```python
from build123d import *

# Parameters (mm, degrees)
EXTRUDE_START   = 4.5
EXTRUDE_1_DEPTH = 3
SKETCH_3_R      = 2.5
EXTRUDE_2_DEPTH = 4.5
SKETCH_6_R      = 3
EXTRUDE_3_DEPTH = 0.5
FILLET_1_R      = 3


with BuildPart() as part:
    # Эскиз2 → Бобышка-Вытянуть1 (new body)
    with BuildSketch(Plane.XY.offset(EXTRUDE_START)):
        with BuildLine():
            ThreePointArc((9, 5.196152423), (0, 0), (9, -5.196152423))
            ThreePointArc((9, -5.196152423), (12, -4.392304845), (15, -5.196152423))
            ThreePointArc((15, -5.196152423), (24, 0), (15, 5.196152423))
            ThreePointArc((15, 5.196152423), (12, 4.392304845), (9, 5.196152423))
        make_face()
    extrude(amount=EXTRUDE_1_DEPTH)

    # Эскиз3 → Бобышка-Вытянуть2 (add)
    with BuildSketch(Plane(origin=(0, 0, 4.5), x_dir=(-1, 0, 0), z_dir=(0, 0, -1))):
        with Locations(Location((-18, 0, 0), (0, 0, 180))):
            Circle(SKETCH_3_R)
        with Locations(Location((-6, 0, 0), (0, 0, 180))):
            Circle(SKETCH_3_R)
    extrude(amount=EXTRUDE_2_DEPTH)

    # Эскиз6 → Бобышка-Вытянуть3 (add)
    with BuildSketch(Plane(origin=(0, 0, 4.5), x_dir=(-1, 0, 0), z_dir=(0, 0, -1))):
        with Locations(Location((-18, 0, 0), (0, 0, 180))):
            Circle(SKETCH_6_R)
        with Locations(Location((-6, 0, 0), (0, 0, 180))):
            Circle(SKETCH_6_R)
    extrude(amount=EXTRUDE_3_DEPTH)

    # Скругление1
    fillet_1_edges = [part.edges().sort_by_distance(p)[0] for p in [
        (0, 0, 7.5),
        (12, 4.392304845, 7.5),
        (24, 0, 7.5),
        (12, -4.392304845, 7.5),
    ]]
    fillet(fillet_1_edges, radius=FILLET_1_R - 0.0001)  # a hair under: the kernel refuses the full size


solid = part.part
```
For this review, take the finished solid that the model builds, in its own axes (mm). A direction names the side the tool comes from. Round coordinates to 2 decimals unless told otherwise and drop trailing zeros. Write each loop counter-clockwise with the first axis right and the second up, starting at its lowest first coordinate (ties: lowest second). Pieces come first, ordered by that corner, then holes. Notation, with made-up numbers: (-5.5, 28.25) -> (8.5, 28.25) arc R21 ccw to (8.5, 66.25) -> close; hole circle Ø2 at (-21.75, -27). An arc over 180 degrees is marked (long way). Use one line per item in the form item = value.
1) Take a section at A-A, the plane z = 2.75. Write out the cut boundary in (x, y).
Found:
outline = circle Ø5 at (6, 0); circle Ø5 at (18, 0)
2) Take a section at D-D, the plane z = 5.25. Write out the cut boundary in (x, y), and give its area (3 significant figures).
Found:
outline = (8.95, -5.11) arc R6.1 cw to (15.05, -5.11) arc R5.9 ccw (long way) to (15.05, 5.11) arc R6.1 cw to (8.95, 5.11) arc R5.9 ccw (long way) to start
area = 232 mm2
3) Tool access review of faces 1 (the flat face through (16, -2, 4)), 2 (the flat face through (6, 0, 0)): name each direction out of +Z, -Z, +X, -X, +Y, -Y from which nothing blocks a thin tool from reaching the whole face with its end or side.
Found:
face_1 = -Z
face_2 = -Z, +X, -X, +Y, -Y
4) Mouldability with a two-part tool opening along X and no side actions: class faces 3 (the cylindrical face through (8.77, 1.15, 4.25)), 4 (the flat face through (12, 0, 7.5)) as +X half, -X half, draft (parallel to the pull), parting line (faces both ways), or undercut.
Found:
face_3 = undercut
face_4 = draft
5) Clearance check with flat-ended pins moving along their axes: pin 1 (2 mm diameter, centred on y = -2.5, z = 2.5, fed in from -X); pin 2 (3 mm diameter, centred on x = 8.5, y = 5, fed in from +Z). State where each tip first meets the part, or that it passes through.
Found:
pin_1 = 4
pin_2 = 7.29
6) Take a section at C-C, the plane z = 6.5. Write out the cut boundary in (x, y), and give its area (3 significant figures).
Found:
outline = (8.62, -4.53) arc R6.76 cw to (15.38, -4.53) arc R5.24 ccw (long way) to (15.38, 4.53) arc R6.76 cw to (8.62, 4.53) arc R5.24 ccw (long way) to start
area = 192 mm2
7) To check wall thickness, follow L1, parallel to Z at x = 5, y = 4; L2, parallel to Z at x = 20.25, y = -1.25; L3, parallel to Y at x = 4, z = 3.5. State the ranges of each line that lie inside material, in increasing order. Write a range as from..to.
Found:
L1 = 4.5..7.28
L2 = 4..7.5
L3 = -1.5..1.5
